Part model, mm, in its own coordinate system. Face numbers are marked on the shaded views. A direction names the side the tool comes from. Give positions to 0.01 mm unless a question says otherwise; leave off trailing zeros. Write each loop counter-clockwise with the first axis right and the second up, starting at its lowest first coordinate (ties: lowest second). Pieces come first, ordered by that corner, then holes.
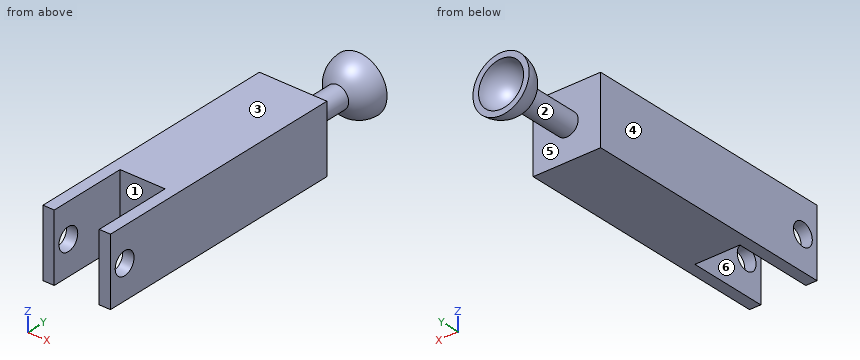
```python
from build123d import *

# Parameters (mm, degrees)
CROQUIS1_W                 = 60
CROQUIS1_H                 = 60
SALIENTE_EXTRUIR1_DEPTH    = 300
CROQUIS2_W                 = 40
CROQUIS2_H                 = 70
CORTAR_EXTRUIR1_DEPTH      = 31
CORTAR_EXTRUIR1_DEPTH_BACK = 31
CROQUIS3_R                 = 10
CORTAR_EXTRUIR2_DEPTH      = 31
CORTAR_EXTRUIR2_DEPTH_BACK = 31


with BuildPart() as part:
    # Croquis1 → Saliente-Extruir1 (new body)
    with BuildSketch(Plane(origin=(0, 0, 0), x_dir=(1, 0, 0), z_dir=(0, 1, 0))):
        Rectangle(CROQUIS1_W, CROQUIS1_H)
    extrude(amount=SALIENTE_EXTRUIR1_DEPTH)

    # Croquis2 → Cortar-Extruir1 (cut, two sides)
    with BuildSketch(Plane.XY) as cortar_extruir1_sk:
        with Locations((0, 35)):
            Rectangle(CROQUIS2_W, CROQUIS2_H)
    extrude(amount=CORTAR_EXTRUIR1_DEPTH, mode=Mode.SUBTRACT)
    extrude(cortar_extruir1_sk.sketch, amount=-CORTAR_EXTRUIR1_DEPTH_BACK, mode=Mode.SUBTRACT)

    # Croquis3 → Cortar-Extruir2 (cut, two sides)
    with BuildSketch(Plane(origin=(0, 0, 0), x_dir=(0, 0, -1), z_dir=(1, 0, 0))) as cortar_extruir2_sk:
        with Locations((0, 15)):
            Circle(CROQUIS3_R)
    extrude(amount=CORTAR_EXTRUIR2_DEPTH, mode=Mode.SUBTRACT)
    extrude(cortar_extruir2_sk.sketch, amount=-CORTAR_EXTRUIR2_DEPTH_BACK, mode=Mode.SUBTRACT)

    # Croquis4 → Cortar-Revolución5 (revolve, cut)
    with BuildSketch(Plane.XY):
        with BuildLine():
            ThreePointArc((-25, 300), (-20.916500663, 286.306936062), (-10, 277.087121525))
            Line((-10, 277.087121525), (-10, 230))
            Line((-10, 230), (-30, 230))
            Line((-30, 230), (-59.400541748, 230))
            Line((-59.400541748, 230), (-59.400541748, 300))
            Line((-59.400541748, 300), (-25, 300))
        make_face()
        with BuildLine():
            Line((0, 300), (-20, 300))
            ThreePointArc((-20, 300), (-14.142135624, 285.857864376), (0, 280))
            Line((0, 280), (0, 300))
        make_face()
    revolve(axis=Axis((0, 300, 0), (0, -1, 0)), mode=Mode.SUBTRACT)


solid = part.part
```
1) Wall check: L1, parallel to Y at x = -26.5, z = 0; L2, parallel to X at y = 42, z = 8.5; L3, parallel to Y at x = -17.5, z = -27.5. Give the ranges that are in metal, low to high.
Answers follow:
L1: y = 0 to 5, 25 to 230
L2: x = -30 to -20, 20 to 30
L3: y = 70 to 230
2) Two-plate mould, pull along X, no slides. Class the marked faces 4, 5 and 6: +X half, -X half, draft (parallel to the pull), parting line (faces both ways), or undercut.
Answers follow:
face 4: -X half
face 5: draft
face 6: undercut
3) 3-axis set-ups, long thin cutter, end or side, ignore diameter. For the marked faces 1, 2 and 3: which of +Z, -Z, +X, -X, +Y, -Y reach the whole face in a straight line?
Answers follow:
face 1: +Z, -Z, -Y
face 2: none
face 3: +Z, +X, -X, +Y, -Y
4) Saw through at A-A, the plane y = 44. Write the cut outline in (x, z), then the cut area to 3 significant figures.
Answers follow:
outline: (-30, -30) - (-20, -30) - (-20, 30) - (-30, 30) - close; (20, -30) - (30, -30) - (30, 30) - (20, 30) - close
area: 1,200 mm2
5) Saw through at B-B, the plane z = 0. Write the cut outline in (x, y).
Answers follow:
outline: (-30, 0) - (-20, 0) - (-20, 5) - (-30, 5) - close; (-30, 25) - (-20, 25) - (-20, 70) - (20, 70) - (20, 25) - (30, 25) - (30, 230) - (10, 230) - (10, 277.09) arc R25 ccw to (25, 300) - (20, 300) arc R20 cw to (-20, 300) - (-25, 300) arc R25 ccw to (-10, 277.09) - (-10, 230) - (-30, 230) - close; (20, 0) - (30, 0) - (30, 5) - (20, 5) - close
6) Pin check, flat tips, straight feed: pin 1 Ø8 at (x, y) = (-12, 268.5) entering from +Z; pin 2 Ø5 at (x, z) = (-14, 6.5) entering from -Y; pin 3 Ø5 at (x, z) = (-19, -17) entering from +Y; pin 4 Ø12 at (y, z) = (15, 0) entering from +X. Stop position of each tip, or through.
Answers follow:
pin 1: stops at z = 6
pin 2: stops at y = 70
pin 3: stops at y = 300
pin 4: passes through
7) Saw through at C-C, the plane x = 0. Write the cut outline in (y, z), then the cut area to 3 significant figures.
Answers follow:
outline: (70, -30) - (230, -30) - (230, -10) - (277.09, -10) arc R25 ccw to (300, -25) - (300, -20) arc R20 cw to (300, 20) - (300, 25) arc R25 ccw to (277.09, 10) - (230, 10) - (230, 30) - (70, 30) - close
area: 10,900 mm2
8) Saw through at D-D, the plane y = 266.5. Write the cut outline in (x, z).
Answers follow:
outline: circle Ø20 at (0, 0)
